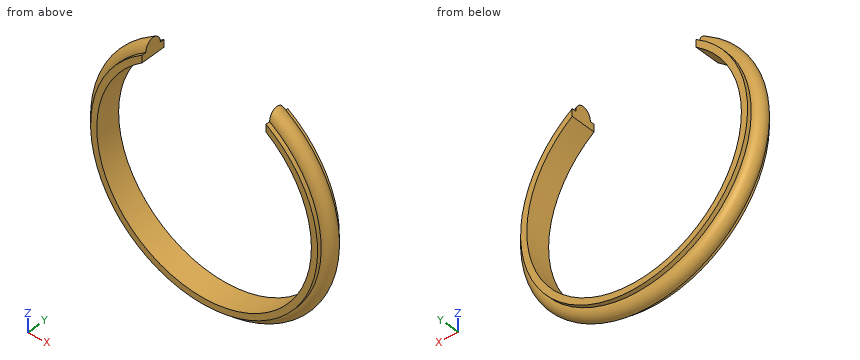
```python
from build123d import *

# Parameters (mm, degrees)
SKETCH3_W          = 30
SKETCH3_H          = 6
CUT_EXTRUDE1_DEPTH = 42.827024898


with BuildPart() as part:
    # Sketch1 → Revolve1 (revolve)
    with BuildSketch(Plane.XY, mode=Mode.PRIVATE) as revolve1_sk:
        with BuildLine():
            Line((-26, -3), (-26, 3))
            Line((-26, 3), (-27.5, 3))
            Line((-27.5, 3), (-27.5, 2))
            ThreePointArc((-27.5, 2), (-29.5, 0), (-27.5, -2))
            Line((-27.5, -2), (-27.5, -3))
            Line((-27.5, -3), (-26, -3))
        make_face()
    revolve(revolve1_sk.sketch.rotate(Axis((0, 27.580200319, 0), (0, -1, 0)), 270), axis=Axis((0, 27.580200319, 0), (0, -1, 0)))

    # Sketch3 → Cut-Extrude1 (cut, through all)
    with BuildSketch(Plane.XY):
        Rectangle(SKETCH3_W, SKETCH3_H)
    extrude(amount=CUT_EXTRUDE1_DEPTH, mode=Mode.SUBTRACT)


solid = part.part
```
Here's how the part is built. I have some questions about the finished solid (model axes, mm). Coordinates: 2 decimals unless noted, no trailing zeros. Order: outer loops, then holes, each group sorted by start corner. A loop starts at its lowest first (then second) coordinate and runs counter-clockwise, first axis right, second up. Notation, with made-up numbers: (24, 31.5) - (67, 31.5) arc R13 cw to (67, 49.5) - close; hole circle Ø1 at (-8.75, -37). An arc over 180 degrees is marked (long way). One line per question, with ' | ' between items.
(1) Suppose I cut it at B-B on x = 0. List the corners of the cut face in (y, z) for me, and give its area (3 significant figures).
Report:
outline: (-3, -27.5) - (-2, -27.5) arc R2 ccw to (2, -27.5) - (3, -27.5) - (3, -26) - (-3, -26) - close | area: 15.3 mm2
(2) Suppose I cut it at A-A on z = 0. List the corners of the cut face in (x, y) for me, and give its area (3 significant figures).
Report:
outline: (-27.5, -3) - (-26, -3) - (-26, 3) - (-27.5, 3) - (-27.5, 2) arc R2 ccw to (-27.5, -2) - close; (26, -3) - (27.5, -3) - (27.5, -2) arc R2 ccw to (27.5, 2) - (27.5, 3) - (26, 3) - close | area: 30.6 mm2
(3) If I drill on L1, parallel to X at y = -2.5, z = -0.5; L2, parallel to X at y = 0.15, z = 0; L3, parallel to Z at x = 17, y = -1.25, over which ranges is the centre line in solid material (lowest first)?
Report:
L1: x = -27.5 to -26, 26 to 27.5 | L2: x = -29.49 to -26, 26 to 29.49 | L3: z = -23.57 to -19.67, 19.67 to 23.57
(4) Will these pins go through, and if not, where does the flat tip stop? pin 1 (2 mm diameter, centred on y = -1, z = -3.5, fed in from +X); pin 2 (2 mm diameter, centred on x = 6, y = -1, fed in from -Z); pin 3 (1 mm diameter, centred on y = 1.5, z = -2, fed in from -X).
Report:
pin 1: stops at x = 29.35 | pin 2: stops at z = -29 | pin 3: stops at x = -29.17
